Autodesk Inventor part; units mm, degrees
ref_plane "YZ Plane" through (0, 0, 0) normal (1, 0, 0) x (0, 1, 0)
ref_plane "XZ Plane" through (0, 0, 0) normal (0, 1, 0) x (-1, 0, 0)
ref_plane "XY Plane" through (0, 0, 0) normal (0, 0, 1) x (1, 0, 0)
sketch "Sketch7" plane through (0, 0, 0) normal (0, 0, 1) x (1, 0, 0)
  circle A0 centre (0, 0) radius 1.75
  dimension "d19" = 3.5
extrude "Extrusion6" add sketch "Sketch7" along normal blind 9
sketch "Sketch8" plane through (0, 0, 9) normal (0, 0, 1) x (1, 0, 0)
  circle A0 centre (0, 0) radius 5
  dimension "d22" = 10
extrude "Extrusion7" add sketch "Sketch8" along normal blind 10
sketch "Sketch9" plane through (0, 0, 19) normal (0, 0, 1) x (1, 0, 0)
  point P0 (0, 0)
  point P1 (0, 0)
hole "Hole1" at (0, 0, 19) direction (0, 0, -1) diameter 3.242 depth 8
properties part number "Elbow_Parallel_Rod_V1"
The listing builds one solid part. Answer for the finished solid, in the listing's coordinates (mm). A direction names the side the tool comes from. Round coordinates to 2 decimals unless told otherwise and drop trailing zeros. Order: outer loops, then holes, each group sorted by start corner. A loop starts at its lowest first (then second) coordinate and runs counter-clockwise, first axis right, second up. Notation, with made-up numbers: (85.5, 61.5) -> (144.5, 61.5) arc R7 ccw to (144.5, 67.5) -> close; hole circle Ø9 at (5, 53.25). An arc over 180 degrees is marked (long way). Write each question's results on one line, items separated by ' | '. Start each with the question number.
Q1. Find section C-C (z = 11.5). Determine the outline of the cut face in (x, y).
Q2. The mould has two halves that part along X. Classify faces 1 (the cylindrical face through (1.438, -0.748, 14.944)), 2 (the cylindrical face through (1.617, 0.67, 4.437)), 3 (the flat face through (2, 0, 19)): pulls with the +X half, pulls with the -X half, needs draft (parallel to the pull), parting line crosses it, or undercut.
Q3. Which of the six approach directions +Z, -Z, +X, -X, +Y, -Y give full straight-line access (tool end or side, diameter ignored) to faces 4 (the flat face through (2, 0, 9)), 5 (the flat face through (0, 0, 11)), 6 (the flat face through (0, 0, 0))?
Q4. Straight lines are drawn through the part: probe 1 along Y at (x, z) = (0, 13.75); probe 2 along Z at (x, y) = (-4, -0.5); probe 3 along Z at (x, y) = (0.5, 1.5). For each, find the intervals that lie inside material, in ascending order. Write a range as from..to.
Q5. Find section A-A (x = 0). Determine the outline of the cut face in (y, z).
Q6. Find section D-D (y = -4). Determine the outline of the cut face in (x, z).
Q7. Each of these flat-tipped pins is pushed along its axis until it touches: pin 1 (3 mm diameter, centred on y = -3, z = 5, fed in from -X); pin 2 (1 mm diameter, centred on y = -3, z = 14, fed in from +X); pin 3 (1 mm diameter, centred on y = -3, z = 3, fed in from -X); pin 4 (5 mm diameter, centred on x = -1.5, z = 5, fed in from -Y). Where does it stop, or does it pass through?
Worked answers:
1) outline: circle Ø10 at (0, 0); hole circle Ø3.24 at (0, 0)
2) face 1: undercut | face 2: parting line crosses it | face 3: needs draft
3) face 4: -Z | face 5: +Z | face 6: -Z, +X, -X, +Y, -Y
4) probe 1: y = -5..-1.62, 1.62..5 | probe 2: z = 9..19 | probe 3: z = 0..11
5) outline: (-5, 9) -> (-1.75, 9) -> (-1.75, 0) -> (1.75, 0) -> (1.75, 9) -> (5, 9) -> (5, 19) -> (1.62, 19) -> (1.62, 11) -> (-1.62, 11) -> (-1.62, 19) -> (-5, 19) -> close
6) outline: (-3, 9) -> (3, 9) -> (3, 19) -> (-3, 19) -> close
7) pin 1: stops at x = -0.9 | pin 2: stops at x = 4.33 | pin 3: passes through | pin 4: stops at y = -1.75
